```python
from build123d import *

# Parameters (mm, degrees)
BASE_FLANGE1_DEPTH = 39
FILLET1_R          = 7
FILLET2_R          = 3
SKETCH6_R          = 14.15
CUT_EXTRUDE1_DEPTH = 10
SKETCH12_R         = 1.5
CUT_EXTRUDE2_DEPTH = 10
SKETCH13_R         = 1.5
CUT_EXTRUDE3_DEPTH = 10


# Sheet-metal steps are written as plain solids
with BuildPart() as part:
    # Sketch1 → Base-Flange1 (new body)
    with BuildSketch(Plane.XY):
        with BuildLine():
            Line((-31.36010038, -13.579909031), (-31.36010038, 25.420090969))
            ThreePointArc((-31.36010038, 25.420090969), (-30.481420723, 27.541411313), (-28.36010038, 28.420090969))
            Line((-28.36010038, 28.420090969), (-11.36010038, 28.420090969))
            Line((-11.36010038, 28.420090969), (-11.36010038, 26.920090969))
            Line((-11.36010038, 26.920090969), (-28.36010038, 26.920090969))
            ThreePointArc((-28.36010038, 26.920090969), (-29.420760552, 26.480751141), (-29.86010038, 25.420090969))
            Line((-29.86010038, 25.420090969), (-29.86010038, -13.579909031))
            Line((-29.86010038, -13.579909031), (-31.36010038, -13.579909031))
        make_face()
    extrude(amount=BASE_FLANGE1_DEPTH)

    # Fillet1
    fillet1_edges = [part.edges().sort_by_distance(p)[0] for p in [
        (-30.61010038, -13.579909031, 39),
        (-30.61010038, -13.579909031, 0),
    ]]
    fillet(fillet1_edges, radius=FILLET1_R)

    # Fillet2
    fillet2_edges = [part.edges().sort_by_distance(p)[0] for p in [
        (-11.36010038, 27.670090969, 39),
        (-11.36010038, 27.670090969, 0),
    ]]
    fillet(fillet2_edges, radius=FILLET2_R)

    # Sketch6 → Cut-Extrude1 (cut)
    with BuildSketch(Plane.ZY.offset(31.36010038)):
        with Locations((19.5, 5.920090969)):
            Circle(SKETCH6_R)
    extrude(amount=-CUT_EXTRUDE1_DEPTH, mode=Mode.SUBTRACT)

    # Sketch12 → Cut-Extrude2 (cut)
    with BuildSketch(Plane.ZY.offset(31.36010038)):
        with Locations((19.204809579, 21.670090969)):
            Circle(SKETCH12_R)
        with Locations((27.117967884, 19.707930885)):
            Circle(SKETCH12_R)
        with Locations((32.989883957, 14.052071253)):
            Circle(SKETCH12_R)
        with Locations((35.24718263, 6.217995095)):
            Circle(SKETCH12_R)
        with Locations((33.285022545, -1.695163209)):
            Circle(SKETCH12_R)
        with Locations((27.629162914, -7.567079283)):
            Circle(SKETCH12_R)
        with Locations((19.795086756, -9.824377956)):
            Circle(SKETCH12_R)
        with Locations((11.881928451, -7.862217871)):
            Circle(SKETCH12_R)
        with Locations((6.010012378, -2.206358239)):
            Circle(SKETCH12_R)
        with Locations((3.752713705, 5.627717919)):
            Circle(SKETCH12_R)
        with Locations((5.71487379, 13.540876223)):
            Circle(SKETCH12_R)
        with Locations((11.370733421, 19.412792296)):
            Circle(SKETCH12_R)
    extrude(amount=-CUT_EXTRUDE2_DEPTH, mode=Mode.SUBTRACT)

    # Sketch13 → Cut-Extrude3 (cut)
    with BuildSketch(Plane(origin=(0, 28.420090969, 0), x_dir=(1, 0, 0), z_dir=(0, 1, 0))):
        with Locations(Location((-26.002140867, -4, 0), (0, 0, 270))):
            Circle(SKETCH13_R)
        with Locations(Location((-20.002140867, -4, 0), (0, 0, 270))):
            Circle(SKETCH13_R)
        with Locations(Location((-14.002140867, -4, 0), (0, 0, 270))):
            Circle(SKETCH13_R)
        with Locations(Location((-20.002140867, -35, 0), (0, 0, 270))):
            Circle(SKETCH13_R)
        with Locations(Location((-14.002140867, -35, 0), (0, 0, 270))):
            Circle(SKETCH13_R)
        with Locations(Location((-26.002140867, -35, 0), (0, 0, 270))):
            Circle(SKETCH13_R)
    extrude(amount=-CUT_EXTRUDE3_DEPTH, mode=Mode.SUBTRACT)


solid = part.part
```
Work out the finished part from the listing and answer in its coordinate system (mm). Give positions to 0.01 mm unless a question says otherwise; leave off trailing zeros. Loops run counter-clockwise (first coordinate to the right, second up) from the corner with the lowest first, then second, coordinate; pieces in that order, holes last. Notation, with made-up numbers: (34, 60.25) -> (61, 60.25) arc R21 cw to (61, 71.25) -> close; hole circle Ø8 at (-11.5, 88.5). An arc over 180 degrees is marked (long way). Put each result on its own line as item: value. Start each with the question number.
Item 1: The part is cut by section A-A (y = 22.5). Give the vertices of the cut face in (x, z).
Item 2: The part is cut by section D-D (z = 19.5). Give the vertices of the cut face in (x, y), then the cut area to 3 significant figures.
Item 3: Each of these flat-tipped pins is pushed along its axis until it touches: P1, Ø1.5, axis at x = -18.5, z = 30, coming from the -Y side; P2, Ø1.8, axis at y = 5.63, z = 3.75, coming from the -X side; P3, Ø5, axis at y = 19.41, z = 11.37, coming from the +X side. Where does it stop, or does it pass through?
Item 4: The part is cut by section C-C (z = 23.5). Give the vertices of the cut face in (x, y).
Item 5: The mould has two halves that part along Y. Classify faces 1 (the face through (-26.577, 27.681, 5.386)), 2 (the face through (-30.62, -9.03, 27.3)), 3 (the face through (-29.4, 26.5, 19.2)): released by +Y, released by -Y, zero draft, split by the parting line, or undercut.
Item 6: The part is cut by section B-B (x = -25). Give the vertices of the cut face in (y, z), then the cut area to 3 significant figures.
Item 7: Find the intervals of material crossed by L1, parallel to X at y = 19.5, z = 7; L2, parallel to Y at x = -15.5, z = 19; L3, parallel to X at y = 28.15, z = 35, in increasing order. Write a range as [from, to].
Answers below:
1. outline: (-31.36, 0) -> (-29.86, 0) -> (-29.86, 17.96) -> (-31.36, 17.96) -> close; (-31.36, 20.45) -> (-29.86, 20.45) -> (-29.86, 39) -> (-31.36, 39) -> close
2. outline: (-31.36, -13.58) -> (-29.86, -13.58) -> (-29.86, -11.3) -> (-31.36, -11.3) -> close; (-31.36, -8.35) -> (-29.86, -8.35) -> (-29.86, -8.23) -> (-31.36, -8.23) -> close; (-31.36, 20.07) -> (-29.86, 20.07) -> (-29.86, 20.2) -> (-31.36, 20.2) -> close; (-31.36, 23.14) -> (-29.86, 23.14) -> (-29.86, 25.42) arc R1.5 cw to (-28.36, 26.92) -> (-11.36, 26.92) -> (-11.36, 28.42) -> (-28.36, 28.42) arc R3 ccw to (-31.36, 25.42) -> close
2. area: 38.0 mm2
3. P1: y = 26.92
3. P2: through
3. P3: x = -29.86
4. outline: (-31.36, -13.58) -> (-29.86, -13.58) -> (-29.86, -7.65) -> (-31.36, -7.65) -> close; (-31.36, 19.49) -> (-29.86, 19.49) -> (-29.86, 25.42) arc R1.5 cw to (-28.36, 26.92) -> (-11.36, 26.92) -> (-11.36, 28.42) -> (-28.36, 28.42) arc R3 ccw to (-31.36, 25.42) -> close
5. face 1: zero draft
5. face 2: undercut
5. face 3: released by -Y
6. outline: (26.92, 0) -> (28.42, 0) -> (28.42, 2.88) -> (26.92, 2.88) -> close; (26.92, 5.12) -> (28.42, 5.12) -> (28.42, 33.88) -> (26.92, 33.88) -> close; (26.92, 36.12) -> (28.42, 36.12) -> (28.42, 39) -> (26.92, 39) -> close
6. area: 51.8 mm2
7. L1: [-31.36, -29.86]
7. L2: [26.92, 28.42]
7. L3: [-29.6, -27.5], [-24.5, -21.5], [-18.5, -15.5], [-12.5, -11.36]
